from build123d import *

# Parameters (mm, degrees)
BOSS_EXTRUDE5_DEPTH = 8
CUT_EXTRUDE4_REACH  = 91.241
SKETCH6_R           = 2.65
CUT_EXTRUDE5_REACH  = 89.972
SKETCH7_R           = 2.65
CUT_EXTRUDE6_REACH  = 74.553
SKETCH8_R           = 2.65
CUT_EXTRUDE7_REACH  = 91.241
SKETCH10_W          = 9.820508075
SKETCH10_H          = 15
SKETCH10_W_2        = 9.820508076


with BuildPart() as part:
    # Sketch1 → Boss-Extrude5 (new body)
    with BuildSketch(Plane(origin=(0, 0, 0), x_dir=(0, 1, 0), z_dir=(0, 0, 1))):
        Polygon((35, 60.621778265), (30, 51.961524227), (50, 17.320508076), (65, 43.301270189), align=None)
        Polygon((60, 0), (0, 0), (30, 51.961524227), align=None)
        Polygon((60, 0), (20, 0), (35, -25.980762114), (65, -8.660254038), align=None)
        Polygon((-10, 0), (0, 0), (20, 34.641016151), (-10, 34.641016151), align=None)
    extrude(amount=BOSS_EXTRUDE5_DEPTH)

    # Sketch6 → Cut-Extrude4 (cut, up to next)
    with BuildSketch(Plane(origin=(-34.641016151, 0, 0), x_dir=(0, -1, 0), z_dir=(-1, 0, 0)), mode=Mode.PRIVATE) as cut_extrude4_sk1:
        with Locations(Location((5, 4, 0), (0, 0, 90))):
            Circle(SKETCH6_R)
    cut_extrude4_tool1 = extrude(cut_extrude4_sk1.sketch, amount=-CUT_EXTRUDE4_REACH, mode=Mode.PRIVATE) & part.part
    add(cut_extrude4_tool1.solids().sort_by_distance((-34.641016, -5, 4))[0], mode=Mode.SUBTRACT)

    # Sketch7 → Cut-Extrude5 (cut, up to next)
    with BuildSketch(Plane(origin=(17.320508076, 30, 0), x_dir=(-0.8660254037844388, 0.49999999999999967, 0), z_dir=(0.49999999999999967, 0.8660254037844388, 0)), mode=Mode.PRIVATE) as cut_extrude5_sk1:
        with Locations((65, 4)):
            Circle(SKETCH7_R)
    cut_extrude5_tool1 = extrude(cut_extrude5_sk1.sketch, amount=-CUT_EXTRUDE5_REACH, mode=Mode.PRIVATE) & part.part
    add(cut_extrude5_tool1.solids().sort_by_distance((-38.971143, 62.5, 4))[0], mode=Mode.SUBTRACT)

    # Sketch8 → Cut-Extrude6 (cut, up to next)
    with BuildSketch(Plane(origin=(-8.660254038, 15, 0), x_dir=(0.8660254037844385, 0.5000000000000003, 0), z_dir=(0.5000000000000003, -0.8660254037844385, 0)), mode=Mode.PRIVATE) as cut_extrude6_sk1:
        with Locations((35, 4)):
            Circle(SKETCH8_R)
    cut_extrude6_tool1 = extrude(cut_extrude6_sk1.sketch, amount=-CUT_EXTRUDE6_REACH, mode=Mode.PRIVATE) & part.part
    add(cut_extrude6_tool1.solids().sort_by_distance((21.650635, 32.5, 4))[0], mode=Mode.SUBTRACT)

    # Sketch10 → Cut-Extrude7 (cut, up to next)
    with BuildSketch(Plane.XY.offset(8), mode=Mode.PRIVATE) as cut_extrude7_sk1:
        with Locations((-29.730762114, -2.5)):
            Rectangle(SKETCH10_W, SKETCH10_H)
    cut_extrude7_tool1 = extrude(cut_extrude7_sk1.sketch, amount=-CUT_EXTRUDE7_REACH, mode=Mode.PRIVATE) & part.part
    # Sketch10 → Cut-Extrude7 (cut, up to next)
    with BuildSketch(Plane.XY.offset(8), mode=Mode.PRIVATE) as cut_extrude7_sk2:
        with Locations((-4.910254038, -2.5)):
            Rectangle(SKETCH10_W_2, SKETCH10_H)
    cut_extrude7_tool2 = extrude(cut_extrude7_sk2.sketch, amount=-CUT_EXTRUDE7_REACH, mode=Mode.PRIVATE) & part.part
    # Sketch10 → Cut-Extrude7 (cut, up to next)
    with BuildSketch(Plane.XY.offset(8), mode=Mode.PRIVATE) as cut_extrude7_sk3:
        Polygon((-60.621778265, 35), (-55.711524227, 43.504809472), (-42.72114317, 36.004809472), (-47.631397208, 27.5), align=None)
    cut_extrude7_tool3 = extrude(cut_extrude7_sk3.sketch, amount=-CUT_EXTRUDE7_REACH, mode=Mode.PRIVATE) & part.part
    # Sketch10 → Cut-Extrude7 (cut, up to next)
    with BuildSketch(Plane.XY.offset(8), mode=Mode.PRIVATE) as cut_extrude7_sk4:
        Polygon((-43.301270189, 65), (-30.310889132, 57.5), (-35.22114317, 48.995190528), (-48.211524227, 56.495190528), align=None)
    cut_extrude7_tool4 = extrude(cut_extrude7_sk4.sketch, amount=-CUT_EXTRUDE7_REACH, mode=Mode.PRIVATE) & part.part
    # Sketch10 → Cut-Extrude7 (cut, up to next)
    with BuildSketch(Plane.XY.offset(8), mode=Mode.PRIVATE) as cut_extrude7_sk5:
        Polygon((8.660254038, 65), (13.570508076, 56.495190528), (0.580127019, 48.995190528), (-4.330127019, 57.5), align=None)
    cut_extrude7_tool5 = extrude(cut_extrude7_sk5.sketch, amount=-CUT_EXTRUDE7_REACH, mode=Mode.PRIVATE) & part.part
    # Sketch10 → Cut-Extrude7 (cut, up to next)
    with BuildSketch(Plane.XY.offset(8), mode=Mode.PRIVATE) as cut_extrude7_sk6:
        Polygon((25.980762114, 35), (12.990381057, 27.5), (8.080127019, 36.004809472), (21.070508076, 43.504809472), align=None)
    cut_extrude7_tool6 = extrude(cut_extrude7_sk6.sketch, amount=-CUT_EXTRUDE7_REACH, mode=Mode.PRIVATE) & part.part
    add(cut_extrude7_tool1.solids().sort_by_distance((-29.730762, -2.5, 8))[0], mode=Mode.SUBTRACT)
    add(cut_extrude7_tool2.solids().sort_by_distance((-4.910254, -2.5, 8))[0], mode=Mode.SUBTRACT)
    add(cut_extrude7_tool3.solids().sort_by_distance((-51.671461, 35.502405, 8))[0], mode=Mode.SUBTRACT)
    add(cut_extrude7_tool4.solids().sort_by_distance((-39.261207, 56.997595, 8))[0], mode=Mode.SUBTRACT)
    add(cut_extrude7_tool5.solids().sort_by_distance((4.620191, 56.997595, 8))[0], mode=Mode.SUBTRACT)
    add(cut_extrude7_tool6.solids().sort_by_distance((17.030445, 35.502405, 8))[0], mode=Mode.SUBTRACT)


solid = part.part
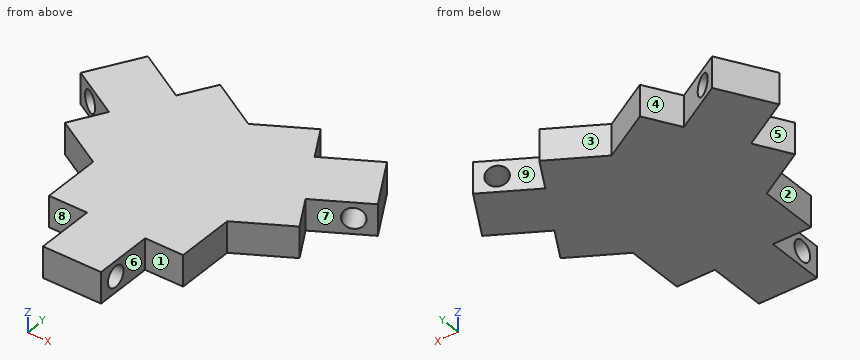
The listing builds one solid part. Answer for the finished solid, in the listing's coordinates (mm). Face numbers are marked on the shaded views. A direction names the side the tool comes from. Round coordinates to 2 decimals unless told otherwise and drop trailing zeros. Write each loop counter-clockwise with the first axis right and the second up, starting at its lowest first coordinate (ties: lowest second). Pieces come first, ordered by that corner, then holes. Notation, with made-up numbers: M 75,25.5 L 94,25.5 A32 ccw 94,61.5 Z; hole C -27,37 d8. An arc over 180 degrees is marked long. Write each question's results on one line, items separated by ' | '. Start each with the question number.
(1) Find the intervals of material crossed by line 1 (X direction, y = 45, z = 5.25); line 2 (Y direction, x = -19, z = 4.5); line 3 (X direction, y = -2.5, z = 7.5), in increasing order.
(2) Determine the mould class of the marked faces 1, 2, 3 and 4 for opening direction X: +X half, -X half, draft (parallel to the pull), parting line (faces both ways), or undercut.
(3) For the marked faces 5, 6, 7, 8 and 9, determine the directions among +Z, -Z, +X, -X, +Y, -Y from which every point of the face is accessible in a straight line to the end or side of a thin tool.
(4) The part is cut by section B-B, the plane z = 4. Give the number of separate pieces and of enclosed holes in the cut face, and give its area (3 significant figures).
(5) The part is cut by section D-D, the plane y = 28.5. Write down the section's boundary in (x, z), and give its area (3 significant figures).
(6) Each of these flat-tipped pins is pushed along its axis until it touches: P1, Ø4, axis at y = 14.5, z = 2, coming from the +X side; P2, Ø2.5, axis at y = -2.5, z = 4.5, coming from the +X side; P3, Ø4, axis at x = -6.5, z = 2.5, coming from the -Y side. Where does it stop, or does it pass through?
(7) The part is cut by section A-A, the plane y = -5. Write down the section's boundary in (x, z).
(8) The part is cut by section C-C, the plane y = 8.5. Write down the section's boundary in (x, z), and give its area (3 significant figures).
Worked answers:
1) line 1: x = -54.85 to -51.77, -46.38 to 11.74, 17.13 to 20.21 | line 2: y = -10 to -7.6, -2.4 to 50.97 | line 3: x = -24.82 to -9.82
2) face 1: draft | face 2: -X half | face 3: undercut | face 4: undercut
3) face 5: +Z, -Z, -X | face 6: +Z, -Z, +X, -Y | face 7: +Z, -Z, +X | face 8: +Z, -Z, -X, -Y | face 9: +Z, -Z, +Y
4) separate pieces: 4 | enclosed holes: 0 | area: 2,510 mm²
5) outline: M -47.05,0 L 12.41,0 L 12.41,8 L -47.05,8 Z | area: 476 mm²
6) P1: stops at x = 0 | P2: stops at x = -9.82 | P3: stops at y = 5
7) outline: M -24.82,0 L -9.82,0 L -9.82,1.35 L -24.82,1.35 Z; M -24.82,6.65 L -9.82,6.65 L -9.82,8 L -24.82,8 Z
8) outline: M -34.64,0 L 0,0 L 0,8 L -34.64,8 Z | area: 277 mm²
